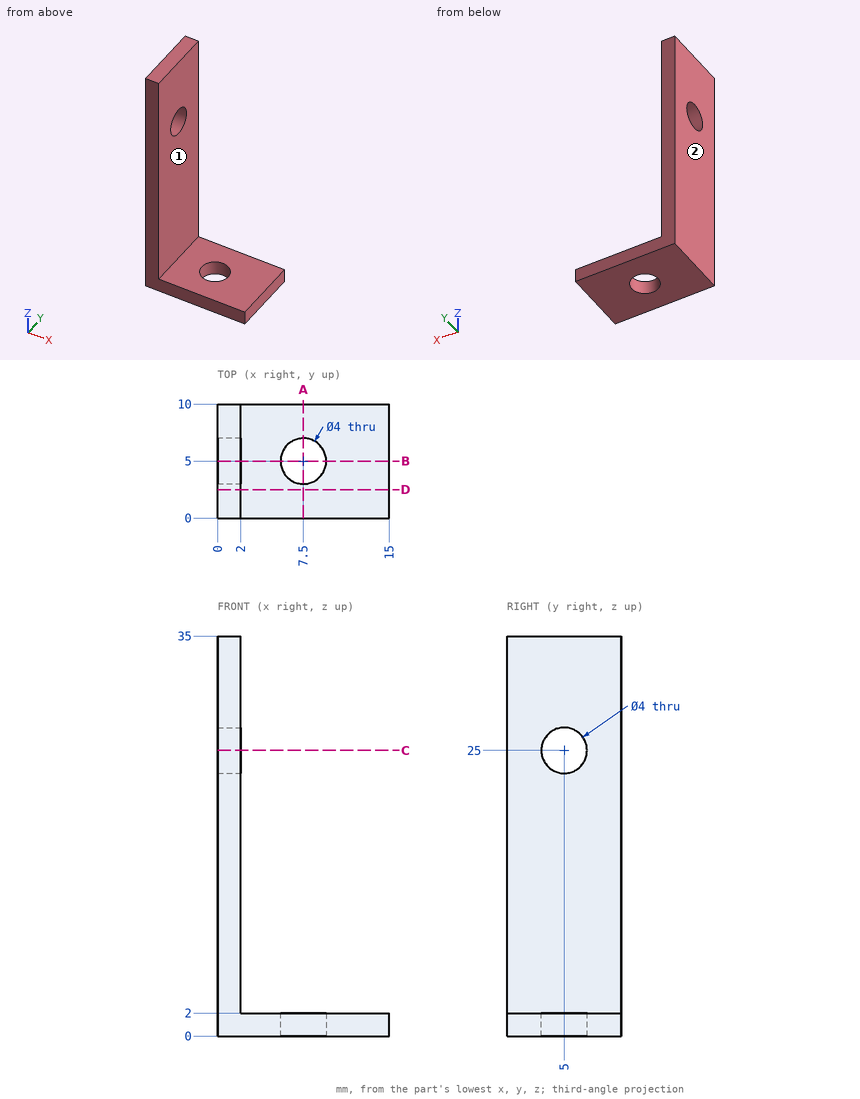
Verification items for this drawing (mm, ordinates from the low corner). A direction names the side the tool comes from. Round coordinates to 2 decimals unless told otherwise and drop trailing zeros. Loops run counter-clockwise (first coordinate to the right, second up) from the corner with the lowest first, then second, coordinate; pieces in that order, holes last. Notation, with made-up numbers: (35.25, 9.25) - (91.25, 9.25) arc R6 ccw to (91.25, 19.25) - close; hole circle Ø2 at (27, -35.5). An arc over 180 degrees is marked (long way). Write item = value, one per line.
Q1. Sectioned sample at C-C on z = 25. Record the boundary of the cut face in (x, y), plus the area to 3 significant figures.
Here are the results:
outline = (0, 0) - (2, 0) - (2, 3) - (0, 3) - close; (0, 7) - (2, 7) - (2, 10) - (0, 10) - close
area = 12.0 mm^2
Q2. Tool access check on the marked faces 1 and 2. Record the directions out of +Z, -Z, +X, -X, +Y, -Y that give a thin tool (end or side, any length) a straight path to the whole face; none if there is none.
Here are the results:
face_1 = +Z, +X, +Y, -Y
face_2 = +Z, -Z, -X, +Y, -Y
Q3. Sectioned sample at B-B on y = 5. Record the boundary of the cut face in (x, z), plus the area to 3 significant figures.
Here are the results:
outline = (0, 0) - (5.5, 0) - (5.5, 2) - (2, 2) - (2, 23) - (0, 23) - close; (0, 27) - (2, 27) - (2, 35) - (0, 35) - close; (9.5, 0) - (15, 0) - (15, 2) - (9.5, 2) - close
area = 80.0 mm^2
Q4. Depth check by flat-ended pin: pin 1 (5 mm diameter, centred on x = 5.5, z = 30.5, fed in from -Y); pin 2 (3 mm diameter, centred on x = 8.5, y = 2.5, fed in from +Z); pin 3 (3 mm diameter, centred on y = 3, z = 15.5, fed in from +X). Enter the tip coordinate at first touch or a pass-through.
Here are the results:
pin_1 = through
pin_2 = 2
pin_3 = 2
Q5. Sectioned sample at D-D on y = 2.5. Record the boundary of the cut face in (x, z), plus the area to 3 significant figures.
Here are the results:
outline = (0, 0) - (15, 0) - (15, 2) - (2, 2) - (2, 35) - (0, 35) - close
area = 96.0 mm^2
Q6. Material ranges on L1, parallel to Y at x = 7.5, z = 0.5; L2, parallel to Z at x = 1, y = 5; L3, parallel to X at y = 1, z = 31.5, recorded low to high.
Here are the results:
L1 = 0 to 3, 7 to 10
L2 = 0 to 23, 27 to 35
L3 = 0 to 2
Q7. Sectioned sample at A-A on x = 7.5. Record the boundary of the cut face in (y, z).
Here are the results:
outline = (0, 0) - (3, 0) - (3, 2) - (0, 2) - close; (7, 0) - (10, 0) - (10, 2) - (7, 2) - close
